from build123d import *

# Parameters (mm, degrees)
F0_W     = 155
F0_H     = 110
F0_W_2   = 82
F0_H_2   = 45
F0_R     = 26.5
F0_R_2   = 24
F0_R_3   = 21.5
F1_DEPTH = 45
F2_W     = 160
F2_H     = 120
F2_W_2   = 155
F2_H_2   = 110
F3_DEPTH = 1
F4_R     = 5
F5_R     = 20
F6_R     = 5.2


with BuildPart() as f1:
    # F0 (on Top) → F1 (new body)
    with BuildSketch(Plane.XY):
        Rectangle(F0_W, F0_H)
        with Locations((-27.5, -25)):
            Rectangle(F0_W_2, F0_H_2, mode=Mode.SUBTRACT)
        with Locations((44.5, -25)):
            Circle(F0_R, mode=Mode.SUBTRACT)
        with Locations((-50, 25)):
            Circle(F0_R_2, mode=Mode.SUBTRACT)
        with Locations((0, 25)):
            Circle(F0_R_2, mode=Mode.SUBTRACT)
        with Locations((50, 25)):
            Circle(F0_R_3, mode=Mode.SUBTRACT)
    extrude(amount=F1_DEPTH)

    # F2 (on face) + F0 (on Top) → F3 (join)
    with BuildSketch(Plane.XY):
        Rectangle(F2_W, F2_H)
        Rectangle(F2_W_2, F2_H_2, mode=Mode.SUBTRACT)
    with BuildSketch(Plane.XY):
        Rectangle(F0_W, F0_H)
        with Locations((-27.5, -25)):
            Rectangle(F0_W_2, F0_H_2, mode=Mode.SUBTRACT)
        with Locations((44.5, -25)):
            Circle(F0_R, mode=Mode.SUBTRACT)
        with Locations((-50, 25)):
            Circle(F0_R_2, mode=Mode.SUBTRACT)
        with Locations((0, 25)):
            Circle(F0_R_2, mode=Mode.SUBTRACT)
        with Locations((50, 25)):
            Circle(F0_R_3, mode=Mode.SUBTRACT)
        with Locations((-27.5, -25)):
            Rectangle(F0_W_2, F0_H_2)
        with Locations((44.5, -25)):
            Circle(F0_R)
        with Locations((0, 25)):
            Circle(F0_R_2)
        with Locations((-50, 25)):
            Circle(F0_R_2)
        with Locations((50, 25)):
            Circle(F0_R_3)
    extrude(amount=-F3_DEPTH)

    # F4
    f4_edges = [f1.edges().sort_by_distance(p)[0] for p in [
        (-80, -60, -0.5),
        (-80, 60, -0.5),
        (80, 60, -0.5),
        (80, -60, -0.5),
    ]]
    fillet(f4_edges, radius=F4_R)

    # F5
    f5_edges = [f1.edges().sort_by_distance(p)[0] for p in [
        (77.5, -55, 22.5),
        (-77.5, -55, 22.5),
        (-77.5, 55, 22.5),
        (77.5, 55, 22.5),
    ]]
    fillet(f5_edges, radius=F5_R)

    # F6
    f6_edges = [f1.edges().sort_by_distance(p)[0] for p in [
        (-68.5, -47.5, 22.5),
        (-68.5, -2.5, 22.5),
        (13.5, -2.5, 22.5),
        (13.5, -47.5, 22.5),
    ]]
    fillet(f6_edges, radius=F6_R)


solid = f1.part
Input: part model. Units: mm. Frame: model coordinates. A direction names the side the tool comes from. Give positions to 0.01 mm unless a question says otherwise; leave off trailing zeros. Loops run counter-clockwise (first coordinate to the right, second up) from the corner with the lowest first, then second, coordinate; pieces in that order, holes last. Notation, with made-up numbers: M 15,70 L 27,70 A27 cw 27,100 Z; hole C -30.75,32.25 d3. An arc over 180 degrees is marked long. Use one line per item in the form item = value.
1. Section query C-C, the plane y = -39.5. Return the cut outline in (x, z).
Numbers:
outline = M -80,-1 L 80,-1 L 80,0 L 76.99,0 L 76.99,45 L 66.68,45 L 66.68,0 L 22.32,0 L 22.32,45 L 13.5,45 L 13.5,0 L -68.5,0 L -68.5,45 L -76.99,45 L -76.99,0 L -80,0 Z
2. Section query A-A, the plane x = -50. Return the cut outline in (y, z), and give its area (3 significant figures).
Numbers:
outline = M -60,-1 L 60,-1 L 60,0 L 55,0 L 55,45 L 49,45 L 49,0 L 1,0 L 1,45 L -2.5,45 L -2.5,0 L -47.5,0 L -47.5,45 L -55,45 L -55,0 L -60,0 Z
area = 885 mm²
3. Section query B-B, the plane z = 17. Return the cut outline in (x, y), and give its area (3 significant figures).
Numbers:
outline = M -77.5,-35 A20 ccw -57.5,-55 L 57.5,-55 A20 ccw 77.5,-35 L 77.5,35 A20 ccw 57.5,55 L -57.5,55 A20 ccw -77.5,35 Z; hole C -50,25 d48; hole M -68.5,-42.3 A5.2 ccw -63.3,-47.5 L 8.3,-47.5 A5.2 ccw 13.5,-42.3 L 13.5,-7.7 A5.2 ccw 8.3,-2.5 L -63.3,-2.5 A5.2 ccw -68.5,-7.7 Z; hole C 0,25 d48; hole C 44.5,-25 d53; hole C 50,25 d43
area = 5,760 mm²
4. Pull-direction query (X, two-part tool) for faces 1 (the face through (-77.5, 0, 22)), 2 (the face through (28.52, 25.95, 22.18)), 3 (the face through (71.797, 48.986, 22.815)); classes: released by +X, released by -X, zero draft, split by the parting line, or undercut.
Numbers:
face_1 = released by -X
face_2 = undercut
face_3 = released by +X
5. Line query: L1, parallel to Y at x = -50, z = 11; L2, parallel to X at y = -26, z = 13; L3, parallel to Y at x = -59.5, z = 9. Output: solid intervals per line, ascending.
Numbers:
L1 = -55 to -47.5, -2.5 to 1, 49 to 55
L2 = -77.5 to -68.5, 13.5 to 18.02, 70.98 to 77.5
L3 = -54.9 to -47.5, -2.5 to 2.96, 47.04 to 54.9
6. First-contact query: pin 1 (10 mm diameter, centred on x = 44, y = 35.5, fed in from +Z); pin 2 (8 mm diameter, centred on x = -60, z = 29.5, fed in from +Y); pin 3 (4 mm diameter, centred on y = -27.5, z = 6.5, fed in from +X). Flat tips, straight axial feed; report the tip coordinate or a pass-through.
Numbers:
pin_1 = 0
pin_2 = 55
pin_3 = 77.5
7. Reachability of faces 4 (the face through (77.5, 0, 22)), 5 (the face through (-1, 55, 22)), 6 (the face through (0, 25, 0)) from +Z, -Z, +X, -X, +Y, -Y: full face, straight path, thin tool, end or side. Return the list, or none.
Numbers:
face_4 = +Z, +X, +Y, -Y
face_5 = +Z, +X, -X, +Y
face_6 = +Z
8. Section query D-D, the plane y = 19.5. Return the cut outline in (x, z).
Numbers:
outline = M -80,-1 L 80,-1 L 80,0 L 77.5,0 L 77.5,45 L 70.78,45 L 70.78,0 L 29.22,0 L 29.22,45 L 23.36,45 L 23.36,0 L -23.36,0 L -23.36,45 L -26.64,45 L -26.64,0 L -73.36,0 L -73.36,45 L -77.5,45 L -77.5,0 L -80,0 Z
